```python
from build123d import *

# Parameters (mm, degrees)
EXTRUDE1_DEPTH = 2
SKETCH2_R      = 1.5
EXTRUDE2_DEPTH = 10
CHAMFER1_SIZE  = 0.307


with BuildPart() as part:
    # Sketch1 → Extrude1 (new body)
    with BuildSketch(Plane.XY):
        Polygon((3.175426481, 0), (1.58771324, 2.75), (-1.58771324, 2.75), (-3.175426481, 0), (-1.58771324, -2.75), (1.58771324, -2.75), align=None)
    extrude(amount=EXTRUDE1_DEPTH)

    # Sketch2 → Extrude2 (add)
    with BuildSketch(Plane.XY.offset(2)):
        Circle(SKETCH2_R)
    extrude(amount=EXTRUDE2_DEPTH)

    # Sketch3 → Cut-Revolve1 (revolve, cut)
    with BuildSketch(Plane(origin=(0, 0, 0), x_dir=(0, 0, -1), z_dir=(1, 0, 0))):
        Polygon((0, 2.75), (0, 102.75), (-57.735026919, 102.75), align=None)
    revolve(axis=Axis((0, 0, 0), (0, 0, -1)), mode=Mode.SUBTRACT)

    # Chamfer1
    chamfer1_edges = [part.edges().sort_by_distance(p)[0] for p in [
        (-1.5, 0, 12),
    ]]
    chamfer(chamfer1_edges, length=CHAMFER1_SIZE)


solid = part.part
```
Work out the finished part from the listing and answer in its coordinate system (mm). A direction names the side the tool comes from. Round coordinates to 2 decimals unless told otherwise and drop trailing zeros. Write each loop counter-clockwise with the first axis right and the second up, starting at its lowest first coordinate (ties: lowest second). Pieces come first, ordered by that corner, then holes.
1) A cutting plane is placed at A-A on z = 10.5. Determine the outline of the cut face in (x, y), and give its area (3 significant figures).
2) Which of the six approach directions +Z, -Z, +X, -X, +Y, -Y give full straight-line access (tool end or side, diameter ignored) to faces 1 (the face through (1.4, 1.3, 2)), 2 (the face through (1.46, -2.51, 0.09))?
3) Flat-ended cylindrical pins translate along their axes: P1, Ø1, axis at y = -0.5, z = 9.5, coming from the -X side; P2, Ø1, axis at x = -1.5, z = 3, coming from the -Y side; P3, Ø1.5, axis at y = 1, z = 4.5, coming from the +X side. Find the tip coordinate at first contact, or state that the pin passes through.
4) Consider probe 1 along Z at (x, y) = (-1.75, -0.75); probe 2 along X at (y, z) = (-0.75, 10.75); probe 3 along Y at (x, z) = (1.75, 0.5). Determine where each line is inside the solid, lowest interval first.
Entries:
1. outline: circle Ø3 at (0, 0)
1. area: 7.07 mm2
2. face 1: +Z
2. face 2: -Z, +X, -Y
3. P1: stops at x = -1.5
3. P2: stops at y = -1.12
3. P3: stops at x = 1.48
4. probe 1: z = 0 to 2
4. probe 2: x = -1.3 to 1.3
4. probe 3: y = -2.47 to 2.47
